Part model, mm, in its own coordinate system. A direction names the side the tool comes from. Round coordinates to 2 decimals unless told otherwise and drop trailing zeros. Order: outer loops, then holes, each group sorted by start corner. A loop starts at its lowest first (then second) coordinate and runs counter-clockwise, first axis right, second up. Notation, with made-up numbers: (36.5, 76) -> (71.5, 76) arc R26 ccw to (71.5, 93) -> close; hole circle Ø8 at (73.5, -0.75). An arc over 180 degrees is marked (long way). Use CSV: the item, a comma, the result in double quotes.
```python
from build123d import *

# Parameters (mm, degrees)
F0_R     = 7.5
F0_W     = 5
F0_H     = 1
F1_DEPTH = 55


with BuildPart() as f1:
    # F0 (on Front) → F1 (new body)
    with BuildSketch(Plane.XZ):
        Polygon((0, 6), (0, 0), (33, 0), (33, 6), (28, 6), (28, 7.833333), (33, 7.833333), (33, 8.833333), (28, 8.833333), (28, 10.166667), (33, 10.166667), (33, 11.166667), (28, 11.166667), (28, 12.5), (33, 12.5), (33, 13.5), (28, 13.5), (28, 14.833333), (33, 14.833333), (33, 15.833333), (28, 15.833333), (28, 17.166667), (33, 17.166667), (33, 18.166667), (28, 18.166667), (28, 19.5), (33, 19.5), (33, 20.5), (28, 20.5), (28, 21.833333), (33, 21.833333), (33, 22.833333), (28, 22.833333), (28, 24.166667), (33, 24.166667), (33, 25.166667), (28, 25.166667), (28, 27), (33, 27), (33, 33), (27, 33), (27, 28), (25.166667, 28), (25.166667, 33), (24.166667, 33), (24.166667, 28), (22.833333, 28), (22.833333, 33), (21.833333, 33), (21.833333, 28), (20.5, 28), (20.5, 33), (19.5, 33), (19.5, 28), (18.166667, 28), (18.166667, 33), (17.166667, 33), (17.166667, 28), (15.833333, 28), (15.833333, 33), (14.833333, 33), (14.833333, 28), (13.5, 28), (13.5, 33), (12.5, 33), (12.5, 28), (11.166667, 28), (11.166667, 33), (10.166667, 33), (10.166667, 28), (8.833333, 28), (8.833333, 33), (7.833333, 33), (7.833333, 28), (6, 28), (6, 33), (0, 33), (0, 27), (5, 27), (5, 25.166667), (0, 25.166667), (0, 24.166667), (5, 24.166667), (5, 22.833333), (0, 22.833333), (0, 21.833333), (5, 21.833333), (5, 20.5), (0, 20.5), (0, 19.5), (5, 19.5), (5, 18.166667), (0, 18.166667), (0, 17.166667), (5, 17.166667), (5, 15.833333), (5, 14.833333), (5, 13.5), (0, 13.5), (0, 12.5), (5, 12.5), (5, 11.166667), (0, 11.166667), (0, 10.166667), (5, 10.166667), (5, 8.833333), (0, 8.833333), (0, 7.833333), (5, 7.833333), (5, 6), align=None)
        with Locations((16.5, 16.5)):
            Circle(F0_R, mode=Mode.SUBTRACT)
        with Locations((2.5, 15.333333)):
            Rectangle(F0_W, F0_H)
    extrude(amount=F1_DEPTH)


solid = f1.part
```
(1) Probe probe 1 along Z at (x, y) = (16.5, -34.5); probe 2 along Z at (x, y) = (6.5, -46.5); probe 3 along X at (y, z) = (-30, 16). List the from-to ranges inside material, lowest first. Write a range as [from, to].
Reply:
probe 1,"[0, 9], [24, 28]"
probe 2,"[0, 28]"
probe 3,"[5, 9.02], [23.98, 28]"
(2) Pull direction X, two halves, no side cores. Call faces 1 (the face through (28, -27, 19)), 2 (the face through (15.833, -27, 30)), 3 (the face through (2, -27, 12.5)): released by +X, released by -X, zero draft, split by the parting line, or undercut.
Reply:
face 1,"released by +X"
face 2,"undercut"
face 3,"zero draft"
(3) Cut at B-B, the plane z = 31.5. State how many separate pieces and enclosed holes the cut face has, then the cut area to 3 significant figures.
Reply:
separate pieces,"10"
enclosed holes,"0"
area,"1,100 mm2"
(4) Cut at C-C, the plane z = 26. Give the cut face in (x, y), then the cut area to 4 significant figures.
Reply:
outline,"(5, -55) -> (28, -55) -> (28, 0) -> (5, 0) -> close"
area,"1,265 mm2"
(5) Which spindle directions (+Z, -Z, +X, -X, +Y, -Y) get a long thin tool onto all of the face, cutting with end or side? Do faces 4 (the face through (20.5, -27, 30)), 5 (the face through (0, -27, 30)), 6 (the face through (30, -27, 12.5)), 7 (the face through (3, -27, 11.167)). Say none if no direction does.
Reply:
face 4,"+Z, +Y, -Y"
face 5,"+Z, -Z, -X, +Y, -Y"
face 6,"+X, +Y, -Y"
face 7,"-X, +Y, -Y"
(6) Cut at A-A, the plane x = 16.5. Give the cut face in (y, z), then the cut area to 3 significant figures.
Reply:
outline,"(-55, 0) -> (0, 0) -> (0, 9) -> (-55, 9) -> close; (-55, 24) -> (0, 24) -> (0, 28) -> (-55, 28) -> close"
area,"715 mm2"
(7) Drop flat-ended pins along their axis: P1, Ø3, axis at x = 7.5, z = 29.5, coming from the +Y side; P2, Ø0.5, axis at y = -23.5, z = 26.5, coming from the -X side; P3, Ø1.5, axis at y = -9, z = 26, coming from the +X side. Give the stop position or say it passes through.
Reply:
P1,"y = 0"
P2,"x = 5"
P3,"x = 28"
